Can you work these out from the model? Positions are in its coordinate system, mm. A direction names the side the tool comes from. Give positions to 0.01 mm unless a question says otherwise; leave off trailing zeros. Write each loop counter-clockwise with the first axis right and the second up, starting at its lowest first coordinate (ties: lowest second). Pieces come first, ordered by that corner, then holes. Notation, with made-up numbers: (-35.5, 20) -> (-28.5, 20) arc R16 cw to (-28.5, 36) -> close; hole circle Ø7 at (48, 88.5). An arc over 180 degrees is marked (long way). One line per item, written item: value.
Autodesk Inventor part; units mm, degrees
ref_plane "Work Plane1" through (0, 0, 12) normal (0, 0, 1) x (1, 0, 0)
ref_plane "YZ Plane" through (0, 0, 0) normal (1, 0, 0) x (0, 1, 0)
ref_plane "XZ Plane" through (0, 0, 0) normal (0, 1, 0) x (-1, 0, 0)
sketch "Sketch1" plane through (0, 0, 0) normal (0, 0, 1) x (1, 0, 0)
  circle A0 centre (0, 0) radius 130
  dimension "d0" = 260
extrude "Extrusion1" add sketch "Sketch1" along normal blind 24
ref_plane "Work Plane1" through (0, 0, 12) normal (0, 0, 1) x (1, 0, 0)
sketch "Sketch3" plane through (0, 0, 12) normal (0, 0, 1) x (1, 0, 0)
  circle A0 centre (0, 0) radius 127.5
  dimension "d4" = 255
extrude "Extrusion2" cut sketch "Sketch3" along normal mid plane 16.5
sketch "Sketch4" plane through (0, 0, 24) normal (0, 0, 1) x (1, 0, 0)
  circle A0 centre (0, 0) radius 12.5
  dimension "d7" = 25
extrude "Extrusion3" cut sketch "Sketch4" against normal blind 5
sketch "Sketch5" plane through (0, 0, 24) normal (0, 0, 1) x (1, 0, 0)
  line L0 (0, 0) -> (91.9239, 91.9239)
  circle A0 centre (0, 0) radius 130
  line L1 (0, 0) -> (130, 0) construction
  line L2 (91.9239, 91.9239) -> (-91.9239, 91.9239)
  arc A1 (91.9239, 91.9239) -> (-91.9239, 91.9239) centre (0, 0) ccw
  dimension "d10" = 45
extrude "Extrusion4" cut sketch "Sketch5" against normal through all contours L2 A0 picked at (-17.7846, 107.7382)
mirror "Mirror1" about plane through (0, 0, 0) normal (0, 1, 0) of "Extrusion4"
sketch "Sketch8" plane through (0, 0, 0) normal (0, 0, -1) x (-1, 0, 0)
  line L0 (91.9239, 91.9239) -> (-91.9239, 91.9239)
  line L1 (-91.9239, 91.9239) -> (91.9239, 91.9239)
  arc A0 (91.9239, -91.9239) -> (91.9239, 91.9239) centre (0, 0) ccw
  arc A1 (91.9239, -91.9239) -> (91.9239, 91.9239) centre (91.9239, 0) ccw
  line L2 (91.9239, -91.9239) -> (-91.9239, -91.9239)
  arc A2 (-91.9239, 91.9239) -> (-91.9239, -91.9239) centre (0, 0) ccw
  arc A3 (-91.9239, 91.9239) -> (-91.9239, -91.9239) centre (-91.9239, 0) ccw
  dimension "d15" = 183.8478
  dimension "d16" = 183.8478
extrude "Extrusion5" cut sketch "Sketch8" against normal blind 3.75
sketch "Sketch9" plane through (-91.9239, 91.9239, 24) normal (0, 1, 0) x (1, 0, 0)
  point P0 (91.9239, 24)
properties part number "Gear Container"
1) I need wall thicknesses on L1, parallel to Y at x = 0, z = 23.2; L2, parallel to Z at x = -75.5, y = 54; L3, parallel to X at y = 10, z = 18. Which ranges of each line are inside material? Lowest first, please.
Answer list:
L1: y = -91.92 to -12.5, 12.5 to 91.92
L2: z = 20.25 to 24
L3: x = -129.61 to -127.11, 127.11 to 129.61
2) Will these pins go through, and if not, where does the flat tip stop? pin 1 (5 mm diameter, centred on y = 14.5, z = 16, fed in from +X); pin 2 (1 mm diameter, centred on y = -8.5, z = 21, fed in from +X); pin 3 (6 mm diameter, centred on y = 50.5, z = 6, fed in from -X).
Answer list:
pin 1: stops at x = 129.44
pin 2: stops at x = 129.75
pin 3: stops at x = -121.01
3) If we section it at C-C (x = 0): Write out the boundary of the cut face in (y, z).
Answer list:
outline: (-91.92, 20.25) -> (-12.5, 20.25) -> (-12.5, 24) -> (-91.92, 24) -> close; (12.5, 20.25) -> (91.92, 20.25) -> (91.92, 24) -> (12.5, 24) -> close
4) We'd pull the mould along X, two halves only. Please class faces 3 (the face through (11.923, 3.755, 22.151)), 4 (the face through (129.992, 1.429, 13.733)), 5 (the face through (-128, 0, 3.75)): released by +X, released by -X, zero draft, split by the parting line, or undercut.
Answer list:
face 3: undercut
face 4: released by +X
face 5: zero draft
5) If we section it at B-B (y = 0): Write out the boundary of the cut face in (x, z).
Answer list:
outline: (-130, 3.75) -> (-127.5, 3.75) -> (-127.5, 20.25) -> (-12.5, 20.25) -> (-12.5, 24) -> (-130, 24) -> close; (12.5, 20.25) -> (127.5, 20.25) -> (127.5, 3.75) -> (130, 3.75) -> (130, 24) -> (12.5, 24) -> close
6) If we section it at D-D (y = 41): Write out the boundary of the cut face in (x, z), and give its area (3 significant figures).
Answer list:
outline: (-123.37, 3.75) -> (-120.73, 3.75) -> (-120.73, 20.25) -> (120.73, 20.25) -> (120.73, 3.75) -> (123.37, 3.75) -> (123.37, 24) -> (-123.37, 24) -> close
area: 1,010 mm^2
7) For faces 1 (the face through (-14, -91.924, 21)), 2 (the face through (127.49, 1.44, 11.88)), which set-ups out of +Z, -Z, +X, -X, +Y, -Y let a thin tool reach every point of the face, with its end or its side?
Answer list:
face 1: +Z, -Z, +X, -X, -Y
face 2: -Z
8) If we section it at A-A (z = 12.75): Write out the boundary of the cut face in (x, y).
Answer list:
outline: (-91.92, -91.92) -> (-88.35, -91.92) arc R127.5 cw to (-88.35, 91.92) -> (-91.92, 91.92) arc R130 ccw to start; (88.35, -91.92) -> (91.92, -91.92) arc R130 ccw to (91.92, 91.92) -> (88.35, 91.92) arc R127.5 cw to start
